Source: three-view drawing plus pictorial views. Frame: mm from the lowest corner of the part. Give positions to 0.01 mm unless a question says otherwise; leave off trailing zeros. Loops run counter-clockwise (first coordinate to the right, second up) from the corner with the lowest first, then second, coordinate; pieces in that order, holes last. Notation, with made-up numbers: M 40,6.5 L 54,6.5 A33 ccw 54,34.5 Z; hole C 15.25,47.5 d8. An arc over 180 degrees is marked long. One line per item, written item: value. Start each with the question number.
(1) Pin query (flat end, axial travel): P1, Ø1.9, axis at x = 185, y = 151, coming from the +Z side. Return the tip coordinate at first contact, or that it passes through.
(2) Section C-C on z = 1.3. State how many separate pieces and enclosed holes the cut face has, plus the area to 3 significant figures.
(3) Ray query, line 1 along Y through (x, z) = (185, 1.2); line 2 along X through (y, z) = (115, 0.85); line 3 along Y through (x, z) = (169, 1.3). Return the intervals inside material, ascending. Write a range as from..to.
(4) Section A-A on x = 98. Output: boundary loops of the cut face in (y, z), plus the area to 3 significant figures.
(5) Section B-B on y = 143.5. Output: boundary loops of the cut face in (x, z).
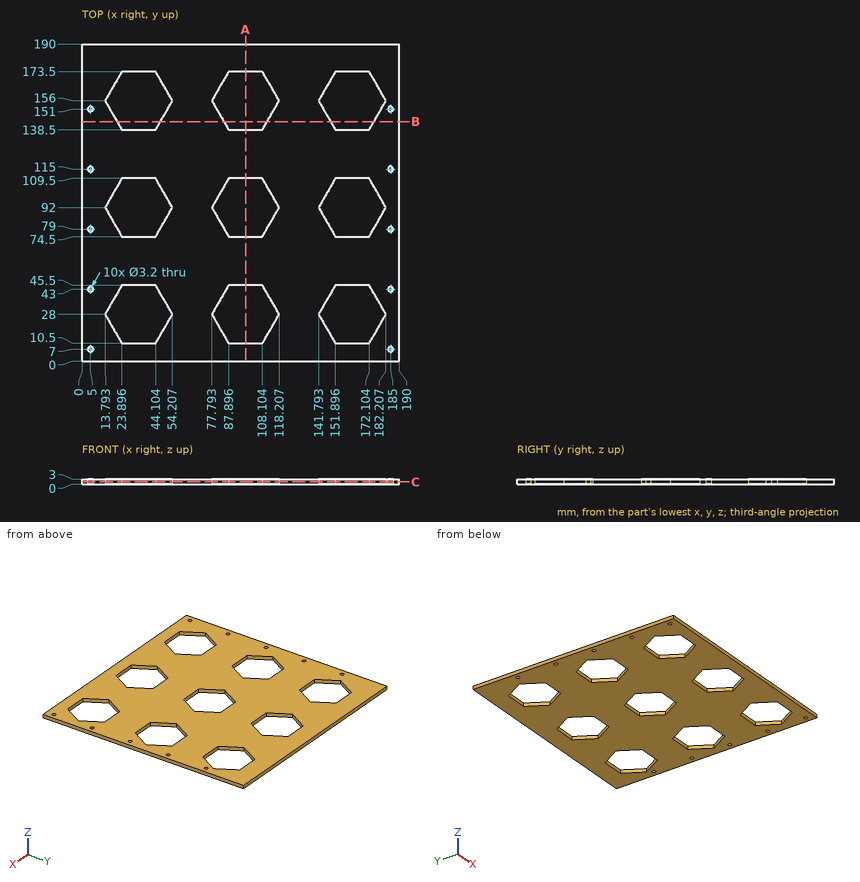
Output values:
1. P1: passes through
2. separate pieces: 1
2. enclosed holes: 19
2. area: 26,500 mm²
3. line 1: y = 0..5.4, 8.6..41.4, 44.6..77.4, 80.6..113.4, 116.6..149.4, 152.6..190
3. line 2: x = 0..3.4, 6.6..183.4, 186.6..190
3. line 3: y = 0..10.5, 45.5..74.5, 109.5..138.5, 173.5..190
4. outline: M 0,0 L 10.5,0 L 10.5,3 L 0,3 Z; M 45.5,0 L 74.5,0 L 74.5,3 L 45.5,3 Z; M 109.5,0 L 138.5,0 L 138.5,3 L 109.5,3 Z; M 173.5,0 L 190,0 L 190,3 L 173.5,3 Z
4. area: 255 mm²
5. outline: M 0,0 L 21.01,0 L 21.01,3 L 0,3 Z; M 46.99,0 L 85.01,0 L 85.01,3 L 46.99,3 Z; M 110.99,0 L 149.01,0 L 149.01,3 L 110.99,3 Z; M 174.99,0 L 190,0 L 190,3 L 174.99,3 Z
